Could you check a few things on this model? Use its own coordinates, in mm. A direction names the side the tool comes from. Give positions to 0.01 mm unless a question says otherwise; leave off trailing zeros. Write each loop counter-clockwise with the first axis right and the second up, starting at its lowest first coordinate (ties: lowest second). Pieces come first, ordered by that corner, then holes. Notation, with made-up numbers: M 75.5,12.5 L 104.5,12.5 A23 ccw 104.5,31.5 Z; hole C 49.25,43 d6. An arc over 180 degrees is marked long. Answer as CSV lines item,"result". Start each with the question number.
Autodesk Inventor part; units mm, degrees
ref_plane "YZ Plane" through (0, 0, 0) normal (1, 0, 0) x (0, 1, 0)
ref_plane "XZ Plane" through (0, 0, 0) normal (0, 1, 0) x (-1, 0, 0)
ref_plane "XY Plane" through (0, 0, 0) normal (0, 0, 1) x (1, 0, 0)
sketch "Sketch1" plane through (0, 0, 0) normal (0, 0, 1) x (1, 0, 0)
  circle A0 centre (0, 0) radius 2.5
  line L0 (2, 1.5) -> (2, -1.5)
  dimension "d0" = 5
  dimension "d1" = 2
extrude "Extrusion1" add sketch "Sketch1" along normal mid plane 35 contours L0 A0 picked at (0.2258, 0.7583)
extrude "Extrusion2" add sketch "Sketch1" along normal mid plane 16 contours A0 L0 picked at (2.0912, -0.3466)
properties part number "CrankShaft"
1. Please list where these lines run through material, in increasing order: line 1 (Y direction, x = -2, z = 5.5); line 2 (X direction, y = -1.9, z = -14); line 3 (X direction, y = -0.45, z = -14).
2. Imagine slicing it at C-C, the plane x = -1.9. Please give me the cut outline in (y, z), plus the area to 3 significant figures.
3. Imagine slicing it at A-A, the plane y = 0. Please give me the cut outline in (x, z).
4. Will these pins go through, and if not, where does the flat tip stop? P1, Ø1.5, axis at x = -2, z = -5, coming from the -Y side; P2, Ø1, axis at x = 1, z = 14, coming from the +Y side; P3, Ø1.5, axis at y = 0, z = -13.5, coming from the +X side.
5. Imagine slicing it at D-D, the plane z = -12.5. Please give me the cut outline in (x, y).
6. On a 3-axis mill with a long thin cutter (end or side, diameter ignored), from which of +Z, -Z, +X, -X, +Y, -Y can I reach the whole of each face in a straight line? I mean faces 1 (the flat face through (2, 0, -13)), 2 (the flat face through (0, 0, 17.5)), 3 (the flat face through (2, 0, 13)). Say none if no direction works.
7. Imagine slicing it at B-B, the plane z = -1. Please give me the cut outline in (x, y), plus the area to 3 significant figures.
Solutions:
1,line 1,"-1.5 to 1.5"
1,line 2,"-1.62 to 1.62"
1,line 3,"-2.46 to 2"
2,outline,"M -1.62,-17.5 L 1.62,-17.5 L 1.62,17.5 L -1.62,17.5 Z"
2,area,"114 mm²"
3,outline,"M -2.5,-17.5 L 2,-17.5 L 2,-8 L 2.5,-8 L 2.5,8 L 2,8 L 2,17.5 L -2.5,17.5 Z"
4,P1,"y = -2.17"
4,P2,"y = 2.45"
4,P3,"x = 2"
5,outline,"M 2,-1.5 L 2,1.5 A2.5 ccw long Z"
6,face 1,"-Z, +X, +Y, -Y"
6,face 2,"+Z, +X, -X, +Y, -Y"
6,face 3,"+Z, +X, +Y, -Y"
7,outline,"C 0,0 d5"
7,area,"19.6 mm²"
